Geometry: final body of the model. Coordinates: model frame, mm. Face numbers are marked on the shaded views. A direction names the side the tool comes from. Round coordinates to 2 decimals unless told otherwise and drop trailing zeros. Loops run counter-clockwise (first coordinate to the right, second up) from the corner with the lowest first, then second, coordinate; pieces in that order, holes last. Notation, with made-up numbers: (-6, -21.75) -> (43, -21.75) arc R23 ccw to (43, -7.75) -> close; hole circle Ø5 at (-19.75, -25). An arc over 180 degrees is marked (long way). Answer in a Markdown table with one row per item.
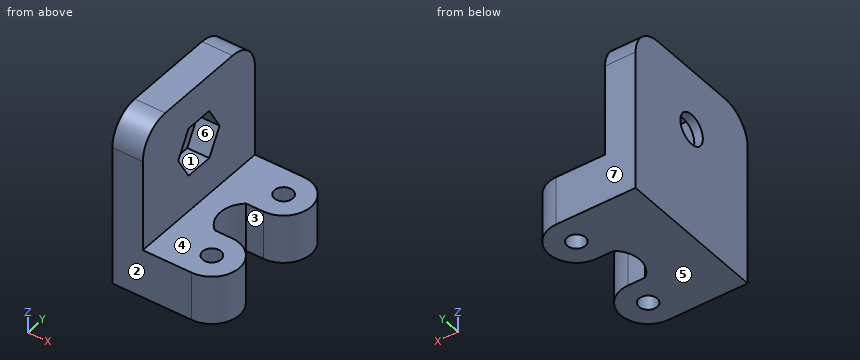
```python
from build123d import *

# Parameters (mm, degrees)
CROQUIS1_R              = 1.5
SALIENTE_EXTRUIR1_DEPTH = 8
CROQUIS2_W              = 5
CROQUIS2_H              = 25
SALIENTE_EXTRUIR2_DEPTH = 20
CROQUIS3_R              = 2.5
CORTAR_EXTRUIR1_DEPTH   = 20
CORTAR_EXTRUIR2_DEPTH   = 3.6
REDONDEO1_R             = 5


with BuildPart() as part:
    # Croquis1 → Saliente-Extruir1 (new body)
    with BuildSketch(Plane.XY):
        with BuildLine():
            Line((-13, 20.5), (0, 20.5))
            ThreePointArc((0, 20.5), (4.5, 16), (0, 11.5))
            Line((0, 11.5), (-2.828427125, 11.5))
            ThreePointArc((-2.828427125, 11.5), (-4.5, 8), (-2.828427125, 4.5))
            Line((-2.828427125, 4.5), (0, 4.5))
            ThreePointArc((0, 4.5), (4.5, 0), (0, -4.5))
            Line((0, -4.5), (-13, -4.5))
            Line((-13, -4.5), (-13, 20.5))
        make_face()
        Circle(CROQUIS1_R, mode=Mode.SUBTRACT)
        with Locations((0, 16)):
            Circle(CROQUIS1_R, mode=Mode.SUBTRACT)
    extrude(amount=SALIENTE_EXTRUIR1_DEPTH)

    # Croquis2 → Saliente-Extruir2 (add)
    with BuildSketch(Plane.XY.offset(8)):
        with Locations((-10.5, 8)):
            Rectangle(CROQUIS2_W, CROQUIS2_H)
    extrude(amount=SALIENTE_EXTRUIR2_DEPTH)

    # Croquis3 → Cortar-Extruir1 (cut)
    with BuildSketch(Plane(origin=(-8, 0, 0), x_dir=(0, 0, -1), z_dir=(1, 0, 0))):
        with Locations((-18, 8)):
            Circle(CROQUIS3_R)
    extrude(amount=-CORTAR_EXTRUIR1_DEPTH, mode=Mode.SUBTRACT)

    # Croquis4 → Cortar-Extruir2 (cut)
    with BuildSketch(Plane(origin=(-8, 0, 0), x_dir=(0, 0, -1), z_dir=(1, 0, 0))):
        Polygon((-18, 3.381197846), (-14, 5.690598923), (-14, 10.309401077), (-18, 12.618802154), (-22, 10.309401077), (-22, 5.690598923), align=None)
    extrude(amount=-CORTAR_EXTRUIR2_DEPTH, mode=Mode.SUBTRACT)

    # Redondeo1
    redondeo1_edges = [part.edges().sort_by_distance(p)[0] for p in [
        (-10.5, -4.5, 28),
        (-10.5, 20.5, 28),
    ]]
    fillet(redondeo1_edges, radius=REDONDEO1_R)


solid = part.part
```
Item 1: Cut plane A-A (z = 6.5). Output: boundary loops of the cut face in (x, y), then the cut area to 3 significant figures.
Answer:
| item | result |
|---|---|
| outline | (-13, -4.5) -> (0, -4.5) arc R4.5 ccw to (0, 4.5) -> (-2.83, 4.5) arc R4.5 cw to (-2.83, 11.5) -> (0, 11.5) arc R4.5 ccw to (0, 20.5) -> (-13, 20.5) -> close; hole circle Ø3 at (0, 0); hole circle Ø3 at (0, 16) |
| area | 347 mm² |
Item 2: Line query: probe 1 along Y at (x, z) = (0, 4); probe 2 along Y at (x, z) = (-12.55, 18); probe 3 along Z at (x, y) = (-9.75, 9.25). Output: solid intervals per line, ascending. Write a range as [from, to].
Answer:
| item | result |
|---|---|
| probe 1 | y = [-4.5, -1.5], [1.5, 4.5], [11.5, 14.5], [17.5, 20.5] |
| probe 2 | y = [-4.5, 5.5], [10.5, 20.5] |
| probe 3 | z = [0, 14], [22, 28] |
Item 3: Draft query along Z for the marked faces 5, 6 and 7. Return one class per face: pulls with the +Z half, pulls with the -Z half, needs draft (parallel to the pull), parting line crosses it, or undercut.
Answer:
| item | result |
|---|---|
| face 5 | pulls with the -Z half |
| face 6 | undercut |
| face 7 | needs draft |
Item 4: Pin query (flat end, axial travel): pin 1 Ø10 at (x, y) = (-4, 8) entering from +Z; pin 2 Ø5 at (x, y) = (0, 0) entering from +Z; pin 3 Ø6 at (x, z) = (-4.5, 24.5) entering from -Y; pin 4 Ø5 at (y, z) = (6.5, 22) entering from +X. Return the tip coordinate at first contact, or that it passes through.
Answer:
| item | result |
|---|---|
| pin 1 | stops at z = 28 |
| pin 2 | stops at z = 8 |
| pin 3 | passes through |
| pin 4 | stops at x = -8 |
Item 5: Reachability of the marked faces 1, 2, 3 and 4 from +Z, -Z, +X, -X, +Y, -Y: full face, straight path, thin tool, end or side. Return the list, or none.
Answer:
| item | result |
|---|---|
| face 1 | +X |
| face 2 | +Z, -Z, +X, -X, -Y |
| face 3 | +Z, -Z, +X |
| face 4 | +Z, +X, +Y, -Y |
Item 6: Cut plane B-B (y = 8). Output: boundary loops of the cut face in (x, z), then the cut area to 3 significant figures.
Answer:
| item | result |
|---|---|
| outline | (-13, 0) -> (-4.5, 0) -> (-4.5, 8) -> (-8, 8) -> (-8, 14) -> (-11.6, 14) -> (-11.6, 15.5) -> (-13, 15.5) -> close; (-13, 20.5) -> (-11.6, 20.5) -> (-11.6, 22) -> (-8, 22) -> (-8, 28) -> (-13, 28) -> close |
| area | 132 mm² |
Item 7: Cut plane D-D (x = -3.25). Output: boundary loops of the cut face in (y, z).
Answer:
| item | result |
|---|---|
| outline | (-4.5, 0) -> (4.89, 0) -> (4.89, 8) -> (-4.5, 8) -> close; (11.11, 0) -> (20.5, 0) -> (20.5, 8) -> (11.11, 8) -> close |
Item 8: Cut plane C-C (x = -11.25). Output: boundary loops of the cut face in (y, z).
Answer:
| item | result |
|---|---|
| outline | (-4.5, 0) -> (20.5, 0) -> (20.5, 23) arc R5 ccw to (15.5, 28) -> (0.5, 28) arc R5 ccw to (-4.5, 23) -> close; hole (3.38, 18) -> (5.69, 14) -> (10.31, 14) -> (12.62, 18) -> (10.31, 22) -> (5.69, 22) -> close |
